For this review, take the finished solid that the model builds, in its own axes (mm). Coordinates: 2 decimals unless noted, no trailing zeros. Order: outer loops, then holes, each group sorted by start corner. A loop starts at its lowest first (then second) coordinate and runs counter-clockwise, first axis right, second up. Notation, with made-up numbers: M 72,75.25 L 83,75.25 A26 cw 83,111.25 Z; hole C 61.25,79 d10. An arc over 180 degrees is marked long. Use one line per item in the form item = value. Start each with the question number.
```python
from build123d import *

# Parameters (mm, degrees)
ESQUISSE1_R        = 4.15
BOSS_EXTRU_1_DEPTH = 15


with BuildPart() as part:
    # Esquisse1 → Boss.-Extru.1 (new body)
    with BuildSketch(Plane(origin=(0, 0, 0), x_dir=(1, 0, 0), z_dir=(0, 1, 0))):
        with BuildLine():
            Line((25, 31.224989992), (25, 95))
            ThreePointArc((25, 95), (0, 120), (-25, 95))
            Line((-25, 95), (-25, 31.224989992))
            ThreePointArc((-25, 31.224989992), (0, 40), (25, 31.224989992))
        make_face()
        with Locations(Location((0, 95, 0), (0, 0, 270))):  # turned: the seam where the file's is
            Circle(ESQUISSE1_R, mode=Mode.SUBTRACT)
    extrude(amount=BOSS_EXTRU_1_DEPTH)


solid = part.part
```
1. The part is to be moulded in two halves that separate along X. For faces 1 (the cylindrical face through (0.55, 7.395, -119.994)), 2 (the cylindrical face through (0.182, 7.395, -99.146)), 3 (the flat face through (0, 15, -76)), 4 (the cylindrical face through (0, 7, -40)), say which applies: pulls with the +X half, pulls with the -X half, needs draft (parallel to the pull), parting line crosses it, or undercut.
2. To check wall thickness, follow line 1 (X direction, y = 5.75, z = -95); line 2 (Z direction, x = 2, y = 8); line 3 (X direction, y = 7.25, z = -104). State the ranges of each line that lie inside material, in increasing order.
3. Consider section D-D, the plane x = -16.5. Write out the cut boundary in (y, z).
4. For pin 1 Ø12 at (x, z) = (-10.5, -51) entering from -Y; pin 2 Ø8 at (x, y) = (-13.5, 12) entering from +Z; pin 3 Ø4 at (x, y) = (13.5, 3.5) entering from +Z; pin 4 Ø6 at (x, y) = (6.5, 2.5) entering from -Z, all flat-tipped, find the tip position at first contact; note any pin that passes through.
5. Consider section A-A, the plane x = 0. Write out the cut boundary in (y, z), plus the area to 3 significant figures.
6. Consider section C-C, the plane z = -105.5. Write out the cut boundary in (x, y).
7. Consider section B-B, the plane y = 9.5. Write out the cut boundary in (x, z), plus the area to 3 significant figures.
Answers follow:
q1.face_1 = parting line crosses it
q1.face_2 = undercut
q1.face_3 = needs draft
q1.face_4 = undercut
q2.line_1 = -25 to -4.15, 4.15 to 25
q2.line_2 = -119.92 to -98.64, -91.36 to -39.95
q2.line_3 = -23.32 to 23.32
q3.outline = M 0,-113.78 L 15,-113.78 L 15,-36.44 L 0,-36.44 Z
q4.pin_1 = 0
q4.pin_2 = -35.97
q4.pin_3 = -36.87
q4.pin_4 = -119.75
q5.outline = M 0,-120 L 15,-120 L 15,-99.15 L 0,-99.15 Z; M 0,-90.85 L 15,-90.85 L 15,-40 L 0,-40 Z
q5.area = 1,080 mm²
q6.outline = M -22.69,0 L 22.69,0 L 22.69,15 L -22.69,15 Z
q7.outline = M -25,-95 A25 ccw 25,-95 L 25,-31.22 A40 cw -25,-31.22 Z; hole C 0,-95 d8.3
q7.area = 3,820 mm²
